```python
from build123d import *

# Parameters (mm, degrees)
SKETCH1_W               = 100
SKETCH1_H               = 75
PLATE_DEPTH             = 5
SKETCH2_R               = 7
BEARING_SUPPORT_DEPTH   = 5.6
SKETCH3_R               = 3.75
BEARING_PIN_DEPTH       = 7
SKETCH4_R               = 1.75
SCREW_THROUGHHOLE_DEPTH = 17.6
FILLET1_R               = 2
FILLET2_R               = 1


with BuildPart() as part:
    # Sketch1 → Plate (new body)
    with BuildSketch(Plane(origin=(0, 0, 0), x_dir=(0, 1, 0), z_dir=(0, 0, 1))):
        with Locations((50, 37.5)):
            Rectangle(SKETCH1_W, SKETCH1_H)
    extrude(amount=PLATE_DEPTH)

    # Sketch2 → Bearing Support (add)
    with BuildSketch(Plane.XY.offset(5)):
        with Locations(Location((-20, 20, 0), (0, 0, 180))):
            Circle(SKETCH2_R)
    bearing_support = extrude(amount=BEARING_SUPPORT_DEPTH)

    # Sketch3 → Bearing Pin (add)
    with BuildSketch(Plane.XY.offset(10.6)):
        with Locations((-20, 20)):
            Circle(SKETCH3_R)
    bearing_pin = extrude(amount=BEARING_PIN_DEPTH)

    # Sketch4 → Screw ThroughHole (cut)
    with BuildSketch(Plane.XY.offset(17.6)):
        with Locations((-20, 20)):
            Circle(SKETCH4_R)
    screw_throughhole = extrude(amount=-SCREW_THROUGHHOLE_DEPTH, mode=Mode.SUBTRACT)

    # Mirror1: Bearing Support, Bearing Pin, Screw ThroughHole across plane
    add(bearing_support.mirror(Plane(origin=(0, 50, 0), x_dir=(0, 0, 1), z_dir=(0, -1, 0))))
    add(bearing_pin.mirror(Plane(origin=(0, 50, 0), x_dir=(0, 0, 1), z_dir=(0, -1, 0))))
    add(screw_throughhole.mirror(Plane(origin=(0, 50, 0), x_dir=(0, 0, 1), z_dir=(0, -1, 0))), mode=Mode.SUBTRACT)

    # Fillet1
    fillet1_edges = [part.edges().sort_by_distance(p)[0] for p in [
        (-37.5, 100, 5),
        (-13, 20, 5),
        (-75, 50, 5),
        (-13, 80, 5),
        (-37.5, 0, 5),
        (-75, 50, 0),
        (-37.5, 100, 0),
        (0, 50, 0),
        (-37.5, 0, 0),
        (0, 50, 5),
    ]]
    fillet(fillet1_edges, radius=FILLET1_R)

    # Fillet2
    fillet2_edges = [part.edges().sort_by_distance(p)[0] for p in [
        (-23.75, 20, 10.6),
        (-23.75, 80, 10.6),
    ]]
    fillet(fillet2_edges, radius=FILLET2_R)


solid = part.part
```
Part model, mm, in its own coordinate system. A direction names the side the tool comes from. Round coordinates to 2 decimals unless told otherwise and drop trailing zeros. Loops run counter-clockwise (first coordinate to the right, second up) from the corner with the lowest first, then second, coordinate; pieces in that order, holes last.
1. Drill centre lines: line 1 along Y through (x, z) = (-20, 13.75); line 2 along X through (y, z) = (80, 14.25); line 3 along Z through (x, y) = (-29, 36.5). Where is each one in solid material? Low to high.
Solutions:
line 1: y = 16.25 to 18.25, 21.75 to 23.75, 76.25 to 78.25, 81.75 to 83.75
line 2: x = -23.75 to -21.75, -18.25 to -16.25
line 3: z = 0 to 5
2. 3-axis set-ups, long thin cutter, end or side, ignore diameter. For faces 5 (the face through (-19.09, 86.94, 8.77)), 6 (the face through (-74.43, 50.7, 0.6)): which of +Z, -Z, +X, -X, +Y, -Y reach the whole face in a straight line?
Solutions:
face 5: +Z
face 6: -Z, -X, +Y, -Y
3. Slice it at C-C (y = 38.5). Give the cut face in (x, z).
Solutions:
outline: (-75, 2) arc R2 ccw to (-73, 0) - (-2, 0) arc R2 ccw to (0, 2) - (0, 3) arc R2 ccw to (-2, 5) - (-73, 5) arc R2 ccw to (-75, 3) - close
4. Two-plate mould, pull along Y, no slides. Class faces 1 (the face through (-38.03, 0.57, 0.6)), 2 (the face through (-38, 49, 0)), 3 (the face through (-21, 25, 10.6)), 4 (the face through (-20.488, 76.282, 14.558)): pulls with the +Y half, pulls with the -Y half, needs draft (parallel to the pull), parting line crosses it, or undercut.
Solutions:
face 1: pulls with the -Y half
face 2: needs draft
face 3: undercut
face 4: undercut
5. Flat gauge pins, fed straight in: pin 1 (6 mm diameter, centred on x = -32.5, y = 19, fed in from +Z); pin 2 (3 mm diameter, centred on x = -20, y = 80, fed in from -Z); pin 3 (1 mm diameter, centred on y = 25.5, z = 3.5, fed in from +X). Where does each tip first touch, or does it go through?
Solutions:
pin 1: stops at z = 5
pin 2: passes through
pin 3: stops at x = 0
6. Slice it at A-A (y = 20). Give the cut face in (x, z).
Solutions:
outline: (-75, 2) arc R2 ccw to (-73, 0) - (-21.75, 0) - (-21.75, 17.6) - (-23.75, 17.6) - (-23.75, 11.6) arc R1 cw to (-24.75, 10.6) - (-27, 10.6) - (-27, 7) arc R2 cw to (-29, 5) - (-73, 5) arc R2 ccw to (-75, 3) - close; (-18.25, 0) - (-2, 0) arc R2 ccw to (0, 2) - (0, 3) arc R2 ccw to (-2, 5) - (-11, 5) arc R2 cw to (-13, 7) - (-13, 10.6) - (-15.25, 10.6) arc R1 cw to (-16.25, 11.6) - (-16.25, 17.6) - (-18.25, 17.6) - close
7. Slice it at B-B (x = -52.5). Give the cut face in (y, z), and give its area (3 significant figures).
Solutions:
outline: (0, 2) arc R2 ccw to (2, 0) - (98, 0) arc R2 ccw to (100, 2) - (100, 3) arc R2 ccw to (98, 5) - (2, 5) arc R2 ccw to (0, 3) - close
area: 497 mm2
8. Slice it at D-D (x = -20). Count the separate pieces of the cut face and the enclosed holes in it, and give its area (3 significant figures).
Solutions:
separate pieces: 3
enclosed holes: 0
area: 639 mm2
